Could you check a few things on this model? Use its own coordinates, in mm. A direction names the side the tool comes from. Give positions to 0.01 mm unless a question says otherwise; leave off trailing zeros. Write each loop counter-clockwise with the first axis right and the second up, starting at its lowest first coordinate (ties: lowest second). Pieces come first, ordered by that corner, then holes. Notation, with made-up numbers: (54.25, 47) - (93.25, 47) arc R18 cw to (93.25, 78) - close; hole circle Ø7 at (88.25, -14.5). An arc over 180 degrees is marked (long way). Answer as a JSON object with one key per item and string values. Group by question number.
```python
from build123d import *

# Parameters (mm, degrees)
F0_W     = 3
F0_H     = 1
F1_DEPTH = 20


with BuildPart() as f1:
    # F0 (on Front) → F1 (new body)
    with BuildSketch(Plane.XZ):
        with BuildLine():
            Line((14.527637, -2.455674), (-11.472363, -2.455674))
            ThreePointArc((-11.472363, -2.455674), (-12.533023, -2.895014), (-12.972363, -3.955674))
            Line((-12.972363, -3.955674), (-12.972363, -9.455674))
            ThreePointArc((-12.972363, -9.455674), (-12.533023, -10.516334), (-11.472363, -10.955674))
            Line((-11.472363, -10.955674), (-8.872363, -10.955674))
            Line((-8.872363, -10.955674), (-8.872363, -11.955674))
            Line((-8.872363, -11.955674), (-7.372363, -11.955674))
            Line((-7.372363, -11.955674), (-7.372363, -10.955674))
            Line((-7.372363, -10.955674), (10.427637, -10.955674))
            Line((10.427637, -10.955674), (10.427637, -11.955674))
            Line((10.427637, -11.955674), (11.927637, -11.955674))
            Line((11.927637, -11.955674), (11.927637, -10.955674))
            Line((11.927637, -10.955674), (14.527637, -10.955674))
            ThreePointArc((14.527637, -10.955674), (15.588297, -10.516334), (16.027637, -9.455674))
            Line((16.027637, -9.455674), (16.027637, -3.955674))
            ThreePointArc((16.027637, -3.955674), (15.588297, -2.895014), (14.527637, -2.455674))
        make_face()
        with Locations((-8.472363, -6.705674)):
            Rectangle(F0_W, F0_H, mode=Mode.SUBTRACT)
        with Locations((-3.472363, -6.705674)):
            Rectangle(F0_W, F0_H, mode=Mode.SUBTRACT)
        with Locations((1.527637, -6.705674)):
            Rectangle(F0_W, F0_H, mode=Mode.SUBTRACT)
        with Locations((6.527637, -6.705674)):
            Rectangle(F0_W, F0_H, mode=Mode.SUBTRACT)
        with Locations((11.527637, -6.705674)):
            Rectangle(F0_W, F0_H, mode=Mode.SUBTRACT)
    extrude(amount=-F1_DEPTH)


solid = f1.part
```
(1) I need wall thicknesses on L1, parallel to X at y = 8.25, z = -6.5; L2, parallel to Z at x = -3, y = 7.5; L3, parallel to Z at x = -7.5, y = 11. Which ranges of each line are inside material? Lowest first, please.
(2) Will these pins go through, and if not, where does the flat tip stop? P1, Ø0.8, axis at y = 5.5, z = -11.5, coming from the +X side; P2, Ø1.3, axis at x = 13.5, y = 10, coming from the -Z side.
(3) If we mould it in two halves opening along X, with no side actions, what happens to faces 1 (the flat face through (-8, 10, -11.956)), 2 (the cylindrical face through (15.577, 9.86, -10.528)), 3 (the flat face through (-4.972, 10, -7)), 4 (the cylindrical face through (-12.545, 9.86, -10.505))? For each: +X half, -X half, draft (parallel to the pull), parting line (faces both ways), or undercut.
(4) I want a section at C-C, the plane x = 8.5. Please give me the cut outline in (y, z), and give its area (3 significant figures).
(5) For faces 5 (the flat face through (10.428, 9.9, -11.4)), 6 (the flat face through (0.028, 10, -7)), 7 (the flat face through (11.928, 9.9, -11.5)), which set-ups out of +Z, -Z, +X, -X, +Y, -Y let a thin tool reach every point of the face, with its end or its side?
(6) I want a section at B-B, the plane y = 8.25. State how many separate pieces and enclosed holes the cut face has, and give its area (3 significant figures).
(7) I want a section at A-A, the plane x = 12.25. Please give me the cut outline in (y, z), and give its area (3 significant figures).
Entries:
{
 "1": {"L1": "-12.97 to -9.97, -6.97 to -4.97, -1.97 to 0.03, 3.03 to 5.03, 8.03 to 10.03, 13.03 to 16.03", "L2": "-10.96 to -7.21, -6.21 to -2.46", "L3": "-11.96 to -7.21, -6.21 to -2.46"},
 "2": {"P1": "x = 11.93", "P2": "z = -10.96"},
 "3": {"face 1": "draft", "face 2": "+X half", "face 3": "undercut", "face 4": "-X half"},
 "4": {"outline": "(0, -10.96) - (20, -10.96) - (20, -2.46) - (0, -2.46) - close", "area": "170 mm^2"},
 "5": {"face 5": "-Z, +Y, -Y", "face 6": "+Y, -Y", "face 7": "-Z, +X, +Y, -Y"},
 "6": {"separate pieces": "1", "enclosed holes": "5", "area": "233 mm^2"},
 "7": {"outline": "(0, -10.96) - (20, -10.96) - (20, -7.21) - (0, -7.21) - close; (0, -6.21) - (20, -6.21) - (20, -2.46) - (0, -2.46) - close", "area": "150 mm^2"}
}
